Could you check a few things on this model? Use its own coordinates, in mm. A direction names the side the tool comes from. Coordinates: 2 decimals unless noted, no trailing zeros. Order: outer loops, then holes, each group sorted by start corner. A loop starts at its lowest first (then second) coordinate and runs counter-clockwise, first axis right, second up. Notation, with made-up numbers: (54.25, 66.25) - (102.25, 66.25) arc R23 ccw to (102.25, 99.25) - close; hole circle Ø7 at (70, -2). An arc over 180 degrees is marked (long way). Answer as a JSON object with one key per item and string values. Group by question number.
(1) Will these pins go through, and if not, where does the flat tip stop? P1, Ø2, axis at y = -9, z = 3, coming from the +X side; P2, Ø2, axis at x = 44, z = 1.5, coming from the -Y side; P3, Ø2, axis at y = -16.5, z = 1.5, coming from the -X side.
(2) Imagine slicing it at C-C, the plane z = 6.75. Write out the boundary of the cut face in (x, y), and give its area (3 significant figures).
(3) Imagine slicing it at B-B, the plane y = -11. Write out the boundary of the cut face in (x, z).
(4) We'd pull the mould along X, two halves only. Please class faces 1 (the cylindrical face through (27.003, -10.369, 2.028)), 2 (the conical face through (23.657, -16.768, 6.028)), 3 (the flat face through (25, 23, 0)): pulls with the +X half, pulls with the -X half, needs draft (parallel to the pull), parting line crosses it, or undercut.
(5) Imagine slicing it at D-D, the plane x = 5. Write out the boundary of the cut face in (y, z).
(6) Please list where these lines run through material, in increasing order: probe 1 along Y at (x, z) = (25, 1.9); probe 2 along Z at (x, y) = (4, 10.5); probe 3 along Y at (x, z) = (46, 2.5).
(7) Imagine slicing it at A-A, the plane x = 25. Write out the boundary of the cut face in (y, z).
(8) Which directions (+Z, -Z, +X, -X, +Y, -Y) give clear straight access to the entire face, cutting with the end or side of a thin tool? Please do faces 4 (the flat face through (30, -11, 2)), 5 (the flat face through (20, -11, 2)), 6 (the flat face through (0, 25, 2)).
from build123d import *

# Parameters (mm, degrees)
BOSS_EXTRUDE1_DEPTH = 4
SKETCH2_R           = 2
BOSS_EXTRUDE2_DEPTH = 4
BOSS_EXTRUDE2_TAPER = 5
SKETCH3_R           = 2.1
CUT_EXTRUDE1_DEPTH  = 4


with BuildPart() as part:
    # Sketch1 → Boss-Extrude1 (new body)
    with BuildSketch(Plane.XY):
        Polygon((0, 0), (20, 0), (20, -22), (30, -22), (30, 0), (50, 0), (50, 50), (0, 50), align=None)
    extrude(amount=BOSS_EXTRUDE1_DEPTH)

    # Sketch2 → Boss-Extrude2 (add)
    with BuildSketch(Plane.XY.offset(4)):
        with Locations((25, -18)):
            Circle(SKETCH2_R)
        with Locations((25, -4)):
            Circle(SKETCH2_R)
    extrude(amount=BOSS_EXTRUDE2_DEPTH, taper=BOSS_EXTRUDE2_TAPER)

    # Sketch3 → Cut-Extrude1 (cut)
    with BuildSketch(Plane.XY.offset(4)):
        with Locations((25, -11)):
            Circle(SKETCH3_R)
    extrude(amount=-CUT_EXTRUDE1_DEPTH, mode=Mode.SUBTRACT)


solid = part.part
Result set:
{
 "1": {"P1": "stops at x = 30", "P2": "stops at y = 0", "P3": "stops at x = 20"},
 "2": {"outline": "circle Ø3.52 at (25, -18); circle Ø3.52 at (25, -4)", "area": "19.4 mm^2"},
 "3": {"outline": "(20, 0) - (22.9, 0) - (22.9, 4) - (20, 4) - close; (27.1, 0) - (30, 0) - (30, 4) - (27.1, 4) - close"},
 "4": {"face 1": "undercut", "face 2": "parting line crosses it", "face 3": "needs draft"},
 "5": {"outline": "(0, 0) - (50, 0) - (50, 4) - (0, 4) - close"},
 "6": {"probe 1": "y = -22 to -13.1, -8.9 to 50", "probe 2": "z = 0 to 4", "probe 3": "y = 0 to 50"},
 "7": {"outline": "(-22, 0) - (-13.1, 0) - (-13.1, 4) - (-16, 4) - (-16.35, 8) - (-19.65, 8) - (-20, 4) - (-22, 4) - close; (-8.9, 0) - (50, 0) - (50, 4) - (-2, 4) - (-2.35, 8) - (-5.65, 8) - (-6, 4) - (-8.9, 4) - close"},
 "8": {"face 4": "+Z, -Z, +X, -Y", "face 5": "+Z, -Z, -X, -Y", "face 6": "+Z, -Z, -X, +Y, -Y"}
}
